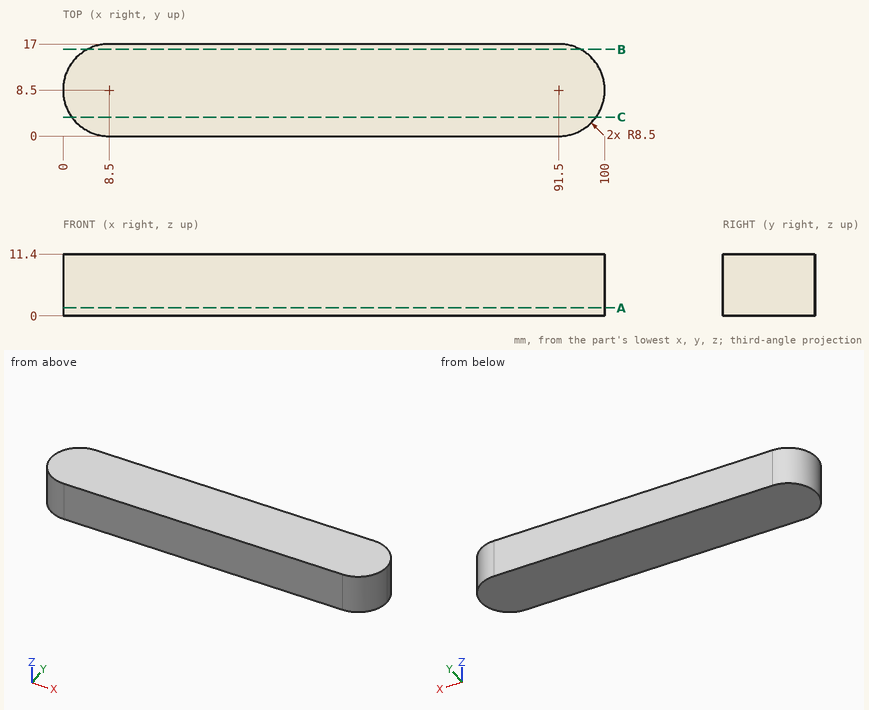
Source: three-view drawing plus pictorial views. Frame: mm from the lowest corner of the part. Round coordinates to 2 decimals unless told otherwise and drop trailing zeros. Loops run counter-clockwise (first coordinate to the right, second up) from the corner with the lowest first, then second, coordinate; pieces in that order, holes last. Notation, with made-up numbers: M 23,-6.75 L 56,-6.75 A17 cw 56,3.25 Z; hole C 5.5,32 d8. An arc over 180 degrees is marked long. Answer as CSV lines item,"result".
Q1. Cut plane C-C (y = 3.5). Return the cut outline in (x, z).
Verdict:
outline,"M 1.63,0 L 98.37,0 L 98.37,11.4 L 1.63,11.4 Z"
Q2. Cut plane A-A (z = 1.5). Return the cut outline in (x, y), plus the area to 3 significant figures.
Verdict:
outline,"M 8.5,0 L 91.5,0 A8.5 ccw 100,8.5 A8.5 ccw 91.5,17 L 8.5,17 A8.5 ccw Z"
area,"1,640 mm^2"
Q3. Cut plane B-B (y = 16). Return the cut outline in (x, z).
Verdict:
outline,"M 4.5,0 L 95.5,0 L 95.5,11.4 L 4.5,11.4 Z"
Q4. Line query: line 1 along X through (y, z) = (8, 3); line 2 along X through (y, z) = (14.75, 0.5); line 3 along Y through (x, z) = (6, 8.5). Output: solid intervals per line, ascending.
Verdict:
line 1,"x = 0.01 to 99.99"
line 2,"x = 2.74 to 97.26"
line 3,"y = 0.38 to 16.62"
Q5. Contact query for flat-ended pins moving along their axis: pin 1 (2 mm diameter, centred on y = 10, z = 2.5, fed in from +X); pin 2 (1.5 mm diameter, centred on y = 9.5, z = 7.5, fed in from -X). Output: stop coordinate, or through.
Verdict:
pin 1,"stops at x = 99.99"
pin 2,"stops at x = 0"
